Model file for the job. Use its own axes, mm. A direction names the side the tool comes from. Coordinates: 2 decimals unless noted, no trailing zeros. Write each loop counter-clockwise with the first axis right and the second up, starting at its lowest first coordinate (ties: lowest second). Pieces come first, ordered by that corner, then holes.
Q1. Which spindle directions (+Z, -Z, +X, -X, +Y, -Y) get a long thin tool onto all of the face, cutting with end or side? Do faces 1 (the flat face through (2, -2, 3)), 2 (the cylindrical face through (-0.54, -2.44, -0.49)), 3 (the flat face through (3.09, -1.75, 1.48)), 4 (the cylindrical face through (0, 1, -2)), 5 (the flat face through (-3.06, -1.8, 1.48)). Say none if no direction does.
Q2. Band-saw the part on B-B, the plane z = 0.75. Write the cut outline in (x, y), plus the area to 3 significant figures.
Q3. Pin check, flat tips, straight feed: P1, Ø2, axis at x = -2.5, z = -2.5, coming from the +Y side; P2, Ø1, axis at y = -1.5, z = -1.5, coming from the +X side; P3, Ø3, axis at y = 0.5, z = -2.5, coming from the -X side. Stop position of each tip, or through.
Q4. Drill centre lines: probe 1 along X at (y, z) = (0, -2.05); probe 2 along Z at (x, y) = (2.25, -1.5). Where is each one in solid material? Low to high.
Q5. Band-saw the part on D-D, the plane z = 3.75. Write the cut outline in (x, y).
Q6. Band-saw the part on C-C, the plane z = -1.5. Write the cut outline in (x, y).
Q7. Pull direction Z, two halves, no side cores. Call faces 6 (the flat face through (-2, -2, -1)), 7 (the flat face through (2, -2, 0)), 8 (the flat face through (3.06, 1.8, 1.48)), 9 (the conical face through (-0.07, 0.32, 0.87)): released by +Z, released by -Z, zero draft, split by the parting line, or undercut.
from build123d import *

# Parameters (mm, degrees)
F0_R      = 2.5
F0_R_2    = 0.2
F1_DEPTH  = 3
F2_SIZE   = 0.54919
F3_DEPTH  = 3.001
F4_DEPTH  = 5
F5_SIZE   = 1.99999
F6_DEPTH  = 1
F7_R      = 3
F7_R_2    = 2.5
F7_R_3    = 0.2
F8_DEPTH  = 4
F9_R      = 1
F9_R_2    = 0.2
F10_DEPTH = 6
F11_SIZE  = 0.79999


# Not quite as in the source:
# - a fillet or chamfer is up to 0.001 mm smaller than in the source, because OpenCascade refuses the exact size


with BuildPart() as f1:
    # F0 (on Top) → F1 (new body)
    with BuildSketch(Plane.XY):
        Polygon((2.0495934556, 3.55), (-2.0495934556, 3.55), (-4.0991869112, 0), (-2.0495934556, -3.55), (2.0495934556, -3.55), (4.0991869112, 0), align=None)
        Circle(F0_R, mode=Mode.SUBTRACT)
        with BuildLine():
            Line((-4.0991869112, 0), (-2.0495934556, 3.55))
            ThreePointArc((-2.0495934556, 3.55), (-3.55, 2.0495934556), (-4.0991869112, 0))
        make_face()
        with BuildLine():
            Line((-2.0495934556, -3.55), (-4.0991869112, 0))
            ThreePointArc((-4.0991869112, 0), (-3.55, -2.0495934556), (-2.0495934556, -3.55))
        make_face()
        with BuildLine():
            ThreePointArc((2.0495934556, 3.55), (0, 4.0991869112), (-2.0495934556, 3.55))
            Line((-2.0495934556, 3.55), (2.0495934556, 3.55))
        make_face()
        with BuildLine():
            ThreePointArc((4.0991869112, 0), (3.55, 2.0495934556), (2.0495934556, 3.55))
            Line((2.0495934556, 3.55), (4.0991869112, 0))
        make_face()
        with BuildLine():
            ThreePointArc((2.0495934556, -3.55), (3.55, -2.0495934556), (4.0991869112, 0))
            Line((4.0991869112, 0), (2.0495934556, -3.55))
        make_face()
        with BuildLine():
            Line((2.0495934556, -3.55), (-2.0495934556, -3.55))
            ThreePointArc((-2.0495934556, -3.55), (0, -4.0991869112), (2.0495934556, -3.55))
        make_face()
        Circle(F0_R)
        Circle(F0_R_2, mode=Mode.SUBTRACT)
    extrude(amount=F1_DEPTH)

    # F2
    f2_edges = [f1.edges().sort_by_distance(p)[0] for p in [
        (2.049593, 3.55, 3),
        (2.049593, 3.55, 0),
    ]]
    chamfer(f2_edges, length=F2_SIZE)

    # F0 (on Top) → F3 (cut, through all)
    with BuildSketch(Plane.XY):
        with BuildLine():
            Line((2.0495934556, -3.55), (-2.0495934556, -3.55))
            ThreePointArc((-2.0495934556, -3.55), (0, -4.0991869112), (2.0495934556, -3.55))
        make_face()
        with BuildLine():
            ThreePointArc((2.0495934556, -3.55), (3.55, -2.0495934556), (4.0991869112, 0))
            Line((4.0991869112, 0), (2.0495934556, -3.55))
        make_face()
        with BuildLine():
            Line((-2.0495934556, -3.55), (-4.0991869112, 0))
            ThreePointArc((-4.0991869112, 0), (-3.55, -2.0495934556), (-2.0495934556, -3.55))
        make_face()
        with BuildLine():
            ThreePointArc((4.0991869112, 0), (3.55, 2.0495934556), (2.0495934556, 3.55))
            Line((2.0495934556, 3.55), (4.0991869112, 0))
        make_face()
        with BuildLine():
            ThreePointArc((2.0495934556, 3.55), (0, 4.0991869112), (-2.0495934556, 3.55))
            Line((-2.0495934556, 3.55), (2.0495934556, 3.55))
        make_face()
        with BuildLine():
            Line((-4.0991869112, 0), (-2.0495934556, 3.55))
            ThreePointArc((-2.0495934556, 3.55), (-3.55, 2.0495934556), (-4.0991869112, 0))
        make_face()
    extrude(amount=F3_DEPTH, mode=Mode.SUBTRACT)

    # F0 (on Top) → F4 (join)
    with BuildSketch(Plane.XY):
        Circle(F0_R)
        Circle(F0_R_2, mode=Mode.SUBTRACT)
    extrude(amount=F4_DEPTH)

    # F5 (size 2 in the source; OpenCascade refuses exactly that, so slightly less here)
    f5_edges = [f1.edges().sort_by_distance(p)[0] for p in [
        (-2.5, 0, 5),
    ]]
    chamfer(f5_edges, length=F5_SIZE)

    # F0 (on Top) → F6 (join)
    with BuildSketch(Plane.XY):
        Circle(F0_R)
        Circle(F0_R_2, mode=Mode.SUBTRACT)
    extrude(amount=-F6_DEPTH)

    # F7 (on face) → F8 (join)
    with BuildSketch(Plane(origin=(0, 0, -1), x_dir=(1, 0, 0), z_dir=(0, 0, -1))):
        Circle(F7_R)
        Circle(F7_R_2, mode=Mode.SUBTRACT)
        Circle(F7_R_2)
        Circle(F7_R_3, mode=Mode.SUBTRACT)
    extrude(amount=F8_DEPTH)

    # F9 (on face) → F10 (cut)
    with BuildSketch(Plane(origin=(0, 0, -5), x_dir=(1, 0, 0), z_dir=(0, 0, -1))):
        Circle(F9_R)
        Circle(F9_R_2, mode=Mode.SUBTRACT)
    extrude(amount=-F10_DEPTH, mode=Mode.SUBTRACT)

    # F11 (size 0.8 in the source; OpenCascade refuses exactly that, so slightly less here)
    f11_edges = [f1.edges().sort_by_distance(p)[0] for p in [
        (-1, 0, 1),
    ]]
    chamfer(f11_edges, length=F11_SIZE)


solid = f1.part
Answer sheet:
1. face 1: +Z
1. face 2: none
1. face 3: +Z, -Z, +X, -Y
1. face 4: -Z
1. face 5: +Z, -Z, -X, -Y
2. outline: (-4.1, 0) - (-2.05, -3.55) - (2.05, -3.55) - (4.1, 0) - (2.05, 3.55) - (-2.05, 3.55) - close; hole circle Ø0.9 at (0, 0)
2. area: 43.0 mm2
3. P1: stops at y = 2.6
3. P2: stops at x = 2.83
3. P3: stops at x = -3
4. probe 1: x = -3 to -1, 1 to 3
4. probe 2: z = -5 to -1, 0 to 3
5. outline: circle Ø3.5 at (0, 0); hole circle Ø0.4 at (0, 0)
6. outline: circle Ø6 at (0, 0); hole circle Ø2 at (0, 0)
7. face 6: undercut
7. face 7: undercut
7. face 8: zero draft
7. face 9: released by -Z
